```python
from build123d import *

# Parameters (mm, degrees)
BOSS_EXTRUDE1_DEPTH   = 50
BOSS_EXTRUDE1_2_DEPTH = 50
BOSS_EXTRUDE2_DEPTH   = 55.499654918
BOSS_EXTRUDE2_START   = 55.499654918
BOSS_EXTRUDE2_2_DEPTH = 0.828043858
BOSS_EXTRUDE2_START_2 = -52
BOSS_EXTRUDE2_3_DEPTH = 4


with BuildPart() as part:
    # airflap → Boss-Extrude1 (new body)
    with BuildSketch(Plane(origin=(0, 0, 0), x_dir=(0, 0, -1), z_dir=(1, 0, 0))):
        with BuildLine():
            ThreePointArc((49.615981669, 11.800608587), (42.648471302, 27.966192012), (30.6, 40.8))
            Line((30.6, 40.8), (30, 40))
            ThreePointArc((30, 40), (41.812226766, 27.417835306), (48.643119283, 11.569224105))
            Line((48.643119283, 11.569224105), (49.615981669, 11.800608587))
        make_face()
    extrude(amount=BOSS_EXTRUDE1_DEPTH)



with BuildPart() as body_2:
    # airflap → Boss-Extrude1 2 (new body)
    with BuildSketch(Plane(origin=(0, 0, 0), x_dir=(0, 0, -1), z_dir=(1, 0, 0))):
        with BuildLine():
            ThreePointArc((30.6, -40.8), (42.648471302, -27.966192012), (49.615981669, -11.800608587))
            Line((49.615981669, -11.800608587), (48.643119283, -11.569224105))
            ThreePointArc((48.643119283, -11.569224105), (41.812226766, -27.417835306), (30, -40))
            Line((30, -40), (30.6, -40.8))
        make_face()
    extrude(amount=BOSS_EXTRUDE1_2_DEPTH)


with BuildPart() as part_1:
    add(part.part)

    add(body_2.part)  # Boss-Extrude2 merges body 2
    # Boss-Extrude2: read off the stored shape, not the designer's step
    # Boss-Extrude2 outline → Boss-Extrude2 (add)
    with BuildSketch(Plane(origin=(0, 0, 0), x_dir=(0, 0, -1), z_dir=(1, 0, 0))):
        with BuildLine():
            ThreePointArc((49.615981669, -11.800608587), (51, 0), (49.615981669, 11.800608587))
            Line((49.615981669, 11.800608587), (48.643119283, 11.569224105))
            ThreePointArc((48.643119283, 11.569224105), (50, 0), (48.643119283, -11.569224105))
            Line((48.643119283, -11.569224105), (49.615981669, -11.800608587))
        make_face()
    extrude(amount=BOSS_EXTRUDE2_DEPTH)

    # Boss-Extrude2 2 outline → Boss-Extrude2 2 (add)
    with BuildSketch(Plane.YZ.offset(BOSS_EXTRUDE2_START)):
        with BuildLine():
            Line((11.800608587, -49.615981669), (11.569224105, -48.643119283))
            ThreePointArc((11.569224105, -48.643119283), (0, -50), (-11.569224105, -48.643119283))
            Line((-11.569224105, -48.643119283), (-11.800608587, -49.615981669))
            ThreePointArc((-11.800608587, -49.615981669), (0, -51), (11.800608587, -49.615981669))
        make_face()
    extrude(amount=BOSS_EXTRUDE2_2_DEPTH)

    # Boss-Extrude2 3 outline → Boss-Extrude2 3 (cut)
    with BuildSketch(Plane.XY.offset(BOSS_EXTRUDE2_START_2)):
        with BuildLine():
            ThreePointArc((56.327698776, 11.800608587), (55.499651286, 0), (56.327698776, -11.800608587))
            Line((56.327698776, -11.800608587), (56.327698776, 11.800608587))
        make_face()
    extrude(amount=BOSS_EXTRUDE2_3_DEPTH, mode=Mode.SUBTRACT)


solid = part_1.part
```
Can you work these out from the model? Positions are in its coordinate system, mm. Give positions to 0.01 mm unless a question says otherwise; leave off trailing zeros. Loops run counter-clockwise (first coordinate to the right, second up) from the corner with the lowest first, then second, coordinate; pieces in that order, holes last. Notation, with made-up numbers: M 85,50 L 118,50 A23 cw 118,88 Z; hole C -2,9.5 d9. An arc over 180 degrees is marked long. Use one line per item in the form item = value. Start each with the question number.
(1) Please list where these lines run through material, in increasing order: line 1 (Y direction, x = 44.5, z = -38.5); line 2 (Y direction, x = 22, z = -42.75); line 3 (Z direction, x = 25.5, y = 0.5).
(2) I want a section at A-A, the plane z = -35. Write out the boundary of the cut face in (x, y), and give its area (3 significant figures).
(3) I want a section at C-C, the plane y = 0. Write out the boundary of the cut face in (x, z).
(4) I want a section at D-D, the plane z = -39.25. Write out the boundary of the cut face in (x, y), and give its area (3 significant figures).
(5) Thinking about a two-plate mould opening in Y: for faces 1 (the flat face through (0, 3.2, -50.6)), 2 (the cylindrical face through (27.77, -0.662, -50.996)), 3 (the cylindrical face through (27.754, 0.649, -49.996)), which applies, released by +Y, released by -Y, zero draft, split by the parting line, or undercut?
(6) I want a section at B-B, the plane x = 30. Write out the boundary of the cut face in (y, z), and give its area (3 significant figures).
(7) I'm going to push flat-ended pins straight in: P1, Ø10, axis at y = 29.5, z = -39, coming from the +X side; P2, Ø10, axis at x = 44.5, z = -47.5, coming from the +Y side; P3, Ø6, axis at x = 18, z = -45, coming from the -Y side. Where does each tip first touch, or does it pass through?
Worked out:
q1.line_1 = -33.45 to -31.9, 31.9 to 33.45
q1.line_2 = -27.81 to -25.93, 25.93 to 27.81
q1.line_3 = -51 to -50
q2.outline = M 0,-37.09 L 50,-37.09 L 50,-35.71 L 0,-35.71 Z; M 0,35.71 L 50,35.71 L 50,37.09 L 0,37.09 Z
q2.area = 139 mm²
q3.outline = M 0,-51 L 55.5,-51 L 55.5,-50 L 0,-50 Z
q4.outline = M 0,-32.56 L 50,-32.56 L 50,-30.97 L 0,-30.97 Z; M 0,30.97 L 50,30.97 L 50,32.56 L 0,32.56 Z
q4.area = 159 mm²
q5.face_1 = zero draft
q5.face_2 = split by the parting line
q5.face_3 = undercut
q6.outline = M -40.8,-30.6 A51 ccw 40.8,-30.6 L 40,-30 A50 cw -40,-30 Z
q6.area = 93.7 mm²
q7.P1 = 50
q7.P2 = 28.19
q7.P3 = -28.93
